Autodesk Inventor part; units mm, degrees
ref_plane "YZ Plane" through (0, 0, 0) normal (1, 0, 0) x (0, 1, 0)
ref_plane "XZ Plane" through (0, 0, 0) normal (0, 1, 0) x (-1, 0, 0)
ref_plane "XY Plane" through (0, 0, 0) normal (0, 0, 1) x (1, 0, 0)
sketch "Sketch1" plane through (0, 0, 0) normal (0, 0, 1) x (1, 0, 0)
  line L0 (0, 0) -> (0, 132.08)
  line L1 (0, 132.08) -> (25.4, 132.08)
  line L2 (0, 66.04) -> (63.5, 66.04)
  line L3 (0, 132.08) -> (0, 66.04)
  line L4 (0, 99.06) -> (31.75, 99.06)
  arc A0 (63.5, 99.06) -> (55.043838, 120.634513) centre (31.75, 99.06) ccw
  line L5 (0, 66.04) -> (0, 0)
  arc A1 (54.194148, 10.562869) -> (63.5, 33.02) centre (31.75, 33.02) ccw
  line L6 (63.5, 28.211314) -> (63.5, 99.06)
  arc A2 (59.079555, 115.220381) -> (25.4, 132.08) centre (28.846947, 96.896052) ccw
  line L7 (0, 0) -> (25.4, 0)
  arc A3 (25.4, 0) -> (63.5, 28.211314) centre (28.813006, 35.223762) ccw
  line L8 (0, 132.08) -> (-25.4, 132.08)
  line L9 (0, 1.27) -> (0, 132.08)
  line L10 (0, 132.08) -> (-25.4, 132.08)
  line L11 (-25.4, 132.08) -> (-25.4, 1.27)
  line L12 (-25.4, 0) -> (0, 0)
  line L13 (0, 0) -> (0, 132.08)
  line L14 (0, 132.08) -> (-25.4, 132.08)
  line L15 (-25.4, 132.08) -> (-25.4, 0)
  dimension "d0" = 132.08
  dimension "d1" = 25.4
  dimension "d2" = 63.5
  dimension "d3" = 25.4
  dimension "d4" = 25.4
sketch "Sketch1 outline for Extrusion1" plane through (0, 0, 0) normal (0, 0, 1) x (1, 0, 0)
  line L0 (-25.4, 0) -> (25.4, 0)
  arc A0 (25.4, 0) -> (63.5, 28.211314) centre (28.813006, 35.223762) ccw
  line L1 (63.5, 28.211314) -> (63.5, 99.06)
  arc A1 (63.5, 99.06) -> (59.079555, 115.220381) centre (31.75, 99.06) ccw
  arc A2 (59.079555, 115.220381) -> (25.4, 132.08) centre (28.846947, 96.896052) ccw
  line L2 (25.4, 132.08) -> (-25.4, 132.08)
  line L3 (-25.4, 132.08) -> (-25.4, 0)
extrude "Extrusion1" add sketch "Sketch1 outline for Extrusion1" along normal blind 787.4
properties part number "Robot Bumper (31 inches)"
CAD build for the part. Positions are in the model's coordinates, mm. Coordinates: 2 decimals unless noted, no trailing zeros. Order: outer loops, then holes, each group sorted by start corner. A loop starts at its lowest first (then second) coordinate and runs counter-clockwise, first axis right, second up.
(1) Pin check, flat tips, straight feed: pin 1 Ø8 at (x, y) = (35.5, 112.5) entering from -Z; pin 2 Ø1.5 at (x, z) = (38, 484.5) entering from -Y; pin 3 Ø8 at (x, z) = (44.5, 554.5) entering from -Y. Stop position of each tip, or through.
Solution:
pin 1: stops at z = 0
pin 2: stops at y = 0.86
pin 3: stops at y = 1.82
(2) Saw through at B-B, the plane x = 47. Write the cut outline in (y, z), and give its area (3 significant figures).
Solution:
outline: (4.87, 0) - (127.23, 0) - (127.23, 787.4) - (4.87, 787.4) - close
area: 96,400 mm2
(3) Drill centre lines: L1, parallel to Y at x = 8.5, z = 649; L2, parallel to Y at x = 51.5, z = 448; L3, parallel to X at y = 6.5, z = 583. Where is each one in solid material? Low to high.
Solution:
L1: y = 0 to 132.08
L2: y = 8.06 to 124.04
L3: x = -25.4 to 49.48
(4) Saw through at A-A, the plane z = 502.5. Write the cut outline in (x, y), and give its area (3 significant figures).
Solution:
outline: (-25.4, 0) - (25.4, 0) arc R35.39 ccw to (63.5, 28.21) - (63.5, 99.06) arc R31.75 ccw to (59.08, 115.22) arc R35.35 ccw to (25.4, 132.08) - (-25.4, 132.08) - close
area: 11,300 mm2
(5) Mould opens along Y. For faces 1 (the face through (50.16, 7, 388.19)), 2 (the face through (63.5, 63, 388)), 3 (the face through (44.423, 128.632, 388.188)) say: released by +Y, released by -Y, zero draft, split by the parting line, or undercut.
Solution:
face 1: released by -Y
face 2: zero draft
face 3: released by +Y
